Read the model definition and answer for the solid it produces. Units are mm, in the model's axes. Give positions to 0.01 mm unless a question says otherwise; leave off trailing zeros. Use a Markdown table: item, result. Add a question column.
Item 1: Consider probe 1 along Z at (x, y) = (3.25, -17.5); probe 2 along Y at (x, z) = (2.75, 10.5); probe 3 along Z at (x, y) = (2.3, -99.5). Determine where each line is inside the solid, lowest interval first. Write a range as [from, to].
Item 2: Each of these flat-tipped pins is pushed along its axis until it touches: P1, Ø1.8, axis at y = -99.48, z = 11.23, coming from the +X side; P2, Ø13, axis at y = -18.41, z = -2.06, coming from the +X side. Where does it stop, or does it pass through?
Item 3: A cutting plane is placed at A-A (x = 3.2). Give the number of separate pieces and of enclosed holes in the cut face, plus the area to 3 significant figures.
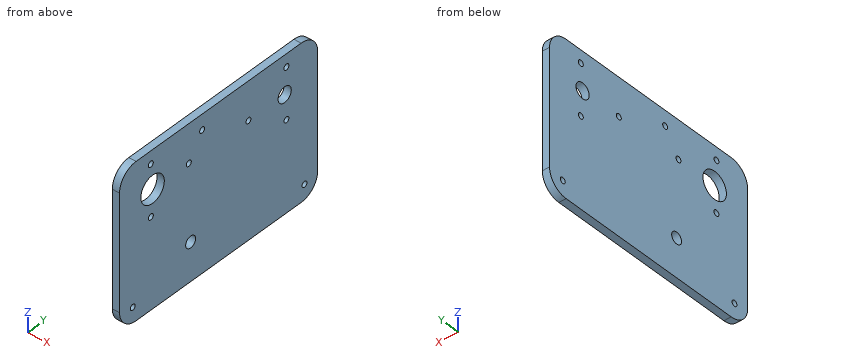
from build123d import *

# Parameters (mm, degrees)
SKETCH1_W           = 80.27017547
SKETCH1_H           = 120
SKETCH1_R           = 4
SKETCH1_R_2         = 7.1
SKETCH1_R_3         = 3
SKETCH1_R_4         = 1.5
BOSS_EXTRUDE1_DEPTH = 3.8
FILLET1_R           = 10


with BuildPart() as part:
    # Sketch1 → Boss-Extrude1 (new body)
    with BuildSketch(Plane(origin=(0, 0, 0), x_dir=(0, 0, -1), z_dir=(1, 0, 0))):
        with Locations((22.195139842, -58.413555688)):
            Rectangle(SKETCH1_W, SKETCH1_H)
        with Locations((2.060052107, -18.413555688)):
            Circle(SKETCH1_R, mode=Mode.SUBTRACT)
        with Locations((2.060052107, -98.413555688)):
            Circle(SKETCH1_R_2, mode=Mode.SUBTRACT)
        with Locations((42.330227577, -75.364196313)):
            Circle(SKETCH1_R_3, mode=Mode.SUBTRACT)
        with Locations((54.330227577, -6.413555688)):
            Circle(SKETCH1_R_4, mode=Mode.SUBTRACT)
        with Locations((54.330227577, -110.413555688)):
            Circle(SKETCH1_R_4, mode=Mode.SUBTRACT)
        with Locations((-9.939947893, -68.413555688)):
            Circle(SKETCH1_R_4, mode=Mode.SUBTRACT)
        with Locations((2.060052107, -76.472881174)):
            Circle(SKETCH1_R_4, mode=Mode.SUBTRACT)
        with Locations((-11.225361719, -99.483892921)):
            Circle(SKETCH1_R_4, mode=Mode.SUBTRACT)
        with Locations((15.345465933, -99.483892921)):
            Circle(SKETCH1_R_4, mode=Mode.SUBTRACT)
        with Locations((15.345465933, -17.343218455)):
            Circle(SKETCH1_R_4, mode=Mode.SUBTRACT)
        with Locations((2.060052107, -40.354230201)):
            Circle(SKETCH1_R_4, mode=Mode.SUBTRACT)
        with Locations((-11.225361719, -17.343218455)):
            Circle(SKETCH1_R_4, mode=Mode.SUBTRACT)
    extrude(amount=BOSS_EXTRUDE1_DEPTH)

    # Fillet1
    fillet1_edges = [part.edges().sort_by_distance(p)[0] for p in [
        (1.9, 1.586444312, 17.939947893),
        (1.9, 1.586444312, -62.330227577),
        (1.9, -118.413555688, -62.330227577),
        (1.9, -118.413555688, 17.939947893),
    ]]
    fillet(fillet1_edges, radius=FILLET1_R)


solid = part.part
Geometry says:
| question | item | result |
|---|---|---|
| 1 | probe 1 | [-62.33, -16.84], [-13.85, -5.95], [1.83, 9.73], [12.72, 17.94] |
| 1 | probe 2 | [-118.08, -100.8], [-98.17, -69.81], [-67.02, -18.66], [-16.03, 1.25] |
| 1 | probe 3 | [-62.33, -16.85], [-13.85, -9.08], [4.96, 9.73], [12.73, 17.94] |
| 2 | P1 | through |
| 2 | P2 | x = 3.8 |
| 3 | separate pieces | 1 |
| 3 | enclosed holes | 12 |
| 3 | area | 9,250 mm² |
